Check sheet for the modelled part. Datum: model origin and axes. Units: mm. Face numbers are marked on the shaded views. A direction names the side the tool comes from. Give positions to 0.01 mm unless a question says otherwise; leave off trailing zeros. Write each loop counter-clockwise with the first axis right and the second up, starting at its lowest first coordinate (ties: lowest second). Pieces come first, ordered by that corner, then holes. Notation, with made-up numbers: (22, 81) -> (53, 81) arc R20 cw to (53, 120) -> close; hole circle Ø4 at (51, 20). An arc over 180 degrees is marked (long way). Answer as a JSON object with one key per item and string values.
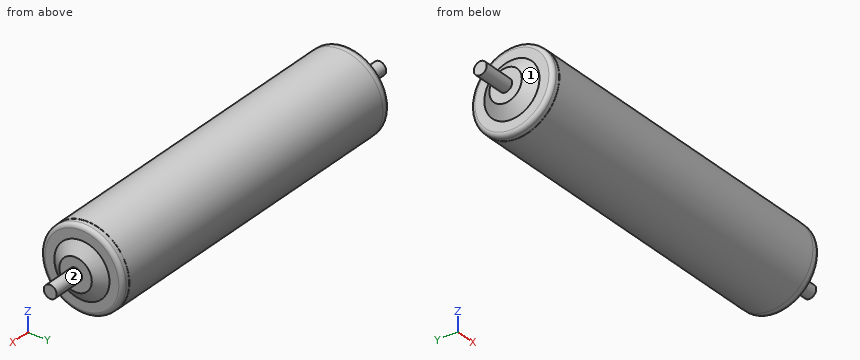
from build123d import *

# Parameters (mm, degrees)
FILLET1_R = 2.5


with BuildPart() as part:
    # Sketch1 → Revolve1 (revolve)
    with BuildSketch(Plane(origin=(0, 0, 0), x_dir=(1, 0, 0), z_dir=(0, 1, 0)), mode=Mode.PRIVATE) as revolve1_sk:
        Polygon((0, 0), (0, -25.4), (100, -25.4), (100, -25.3), (105, -25.3), (105, -17), (110, -10), (110, -4), (130, -4), (130, 0), align=None)
        Polygon((-100, -25.3), (-100, -25.4), (0, -25.4), (0, 0), (-130, 0), (-130, -4), (-110, -4), (-110, -10), (-105, -17), (-105, -25.3), align=None)
    revolve(revolve1_sk.sketch.rotate(Axis((130, 0, 0), (-1, 0, 0)), 180), axis=Axis((130, 0, 0), (-1, 0, 0)))

    # Fillet1
    fillet1_edges = [part.edges().sort_by_distance(p)[0] for p in [
        (105, 0, 25.3),
        (-105, 0, 25.3),
    ]]
    fillet(fillet1_edges, radius=FILLET1_R)


solid = part.part
1. Scan lines: L1, parallel to X at y = -12.5, z = 19.5; L2, parallel to X at y = -9.5, z = 2; L3, parallel to Z at x = -59, y = -1.5. Record each from-to range of solid material in increasing order. Write a range as [from, to].
Determined:
{"L1": "[-104.97, 104.97]", "L2": "[-110, 110]", "L3": "[-25.36, 25.36]"}
2. Access from +Z, -Z, +X, -X, +Y, -Y to the whole of each face (thin tool, end or side, straight path). Record for the marked faces 1 and 2.
Determined:
{"face 1": "-X", "face 2": "+X"}
3. Sectioned sample at C-C, the plane x = 53. Enter the section's corners in (y, z), plus the area to 3 significant figures.
Determined:
{"outline": "circle Ø50.8 at (0, 0)", "area": "2,030 mm^2"}
4. Go/stop test with flat-tipped pins: P1, Ø10, axis at y = -1.5, z = 9, coming from the +X side; P2, Ø1, axis at x = 58, z = 13.5, coming from the +Y side; P3, Ø5, axis at x = 17, z = -11.5, coming from the -Y side; P4, Ø10, axis at y = -2.5, z = 6, coming from the +X side. Record where each tip stops, or that it passes through.
Determined:
{"P1": "x = 110", "P2": "y = 21.82", "P3": "y = -23.75", "P4": "x = 130"}
